Read the model definition and answer for the solid it produces. Units are mm, in the model's axes. Face numbers are marked on the shaded views. A direction names the side the tool comes from. Coordinates: 2 decimals unless noted, no trailing zeros. Loops run counter-clockwise (first coordinate to the right, second up) from the corner with the lowest first, then second, coordinate; pieces in that order, holes last. Notation, with made-up numbers: (32.25, 68.25) -> (40.25, 68.25) arc R34 ccw to (40.25, 106.25) -> close; hole circle Ø3 at (70, -13). An arc over 180 degrees is marked (long way). Answer as a JSON object with one key per item and string values. Group by question number.
1) Section D-D, the plane x = -12.5 is taken. Give the vertices of the cut face in (y, z).
2) Section C-C, the plane z = 1.75 is taken. Give the vertices of the cut face in (x, y).
3) Flat-ended cylindrical pins translate along their axes: P1, Ø5, axis at x = -27, z = 2, coming from the +Y side; P2, Ø6, axis at y = 34, z = 9.5, coming from the +X side; P3, Ø4, axis at x = 14.5, z = 11, coming from the +Y side. Find the tip coordinate at first contact, or state that the pin passes through.
4) Consider probe 1 along Z at (x, y) = (0, 30); probe 2 along Y at (x, z) = (9, 2.5); probe 3 along X at (y, z) = (34.5, 6.25). Determine where each line is inside the solid, lowest interval first. Write a range as [from, to].
5) Which of the six approach directions +Z, -Z, +X, -X, +Y, -Y give full straight-line access (tool end or side, diameter ignored) to the marked faces 1, 2 and 3?
6) Section B-B, the plane y = 0 is taken. Give the vertices of the cut face in (x, z).
7) Section A-A, the plane x = 0 is taken. Give the vertices of the cut face in (y, z), plus the area to 3 significant figures.
8) Determine the mould class of the marked faces 4, 5, 6 and 7 for opening direction Y: released by +Y, released by -Y, zero draft, split by the parting line, or undercut.
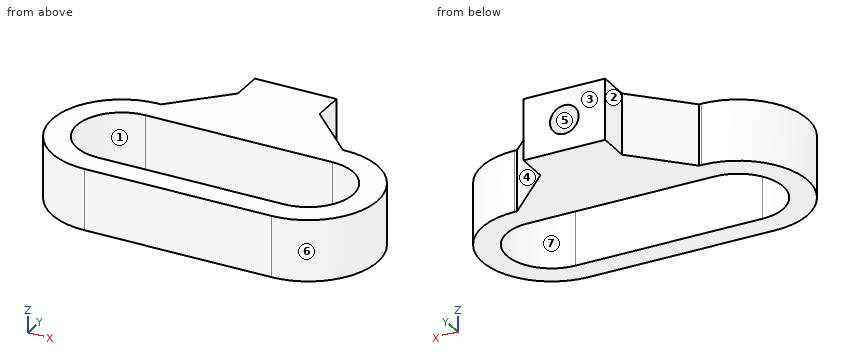
Autodesk Inventor part; units mm, degrees
ref_plane "YZ Plane" through (0, 0, 0) normal (1, 0, 0) x (0, 1, 0)
ref_plane "XZ Plane" through (0, 0, 0) normal (0, 1, 0) x (-1, 0, 0)
ref_plane "XY Plane" through (0, 0, 0) normal (0, 0, 1) x (1, 0, 0)
sketch "Sketch1" plane through (0, 0, 0) normal (0, 0, 1) x (1, 0, 0)
  line L0 (22.86, 0) -> (-22.86, 0) construction
  line L1 (22.86, 11) -> (-22.86, 11)
  line L2 (-22.86, -11) -> (22.86, -11)
  arc A0 (22.86, -11) -> (22.86, 11) centre (22.86, 0) ccw
  arc A1 (-22.86, 11) -> (-22.86, -11) centre (-22.86, 0) ccw
  line L3 (22.86, 0) -> (-22.86, 0) construction
  line L4 (22.86, 17) -> (-22.86, 17)
  line L5 (-22.86, -17) -> (22.86, -17)
  arc A2 (22.86, -17) -> (22.86, 17) centre (22.86, 0) ccw
  arc A3 (-22.86, 17) -> (-22.86, -17) centre (-22.86, 0) ccw
  line L6 (-10, 17) -> (10, 17)
  line L7 (10, 17) -> (10, 37)
  line L8 (10, 37) -> (-10, 37)
  line L9 (-10, 37) -> (-10, 17)
  point P0 (0, 0)
  point P1 (0, 17)
  dimension "d0" = 22
  dimension "d1" = 6
  dimension "d2" = 45.72
  dimension "d3" = 20
  dimension "d4" = 20
extrude "Extrusion1" add sketch "Sketch1" along normal blind 15
sketch "Sketch2" plane through (-10, 37, 0) normal (0, 1, 0) x (1, 0, 0)
  line L0 (-12.86, -15) -> (32.86, -15) construction
  line L1 (10, -15) -> (10, 0) construction
  circle A0 centre (10, -7.5) radius 3.5
  dimension "d7" = 7
extrude "Extrusion2" cut sketch "Sketch2" against normal blind 15
chamfer "Chamfer1" distance 12.25 angle 45 2 edges at (10, 17, 7.5) (-10, 17, 7.5)
properties part number "yoke"
Determined:
{
 "1": {"outline": "(-17, 0) -> (-11, 0) -> (-11, 15) -> (-17, 15) -> close; (11, 0) -> (26.75, 0) -> (26.75, 15) -> (11, 15) -> close"},
 "2": {"outline": "(-22.86, -17) -> (22.86, -17) arc R17 ccw to (22.86, 17) -> (22.25, 17) -> (10, 29.25) -> (10, 37) -> (-10, 37) -> (-10, 29.25) -> (-22.25, 17) -> (-22.86, 17) arc R17 ccw to start; hole (-22.86, -11) -> (22.86, -11) arc R11 ccw to (22.86, 11) -> (-22.86, 11) arc R11 ccw to start"},
 "3": {"P1": "y = 16.92", "P2": "x = 10", "P3": "y = 26.75"},
 "4": {"probe 1": "[0, 4], [11, 15]", "probe 2": "[-17, -11], [11, 37]", "probe 3": "[-10, -3.27], [3.27, 10]"},
 "5": {"face 1": "+Z, -Z", "face 2": "+Z, -Z, -X, +Y", "face 3": "+Z, -Z, +X, -X, +Y"},
 "6": {"outline": "(-39.86, 0) -> (-33.86, 0) -> (-33.86, 15) -> (-39.86, 15) -> close; (33.86, 0) -> (39.86, 0) -> (39.86, 15) -> (33.86, 15) -> close"},
 "7": {"outline": "(-17, 0) -> (-11, 0) -> (-11, 15) -> (-17, 15) -> close; (11, 0) -> (37, 0) -> (37, 4) -> (22, 4) -> (22, 11) -> (37, 11) -> (37, 15) -> (11, 15) -> close", "area": "375 mm²"},
 "8": {"face 4": "released by +Y", "face 5": "zero draft", "face 6": "split by the parting line", "face 7": "undercut"}
}
